from build123d import *

# Parameters (mm, degrees)
SKETCH1_W           = 12.950156288
SKETCH1_H           = 2.985631362
BOSS_EXTRUDE1_DEPTH = 16
FILLET1_R           = 1
SKETCH2_W           = 10.950156288
SKETCH2_H           = 0.272417851
BOSS_EXTRUDE2_DEPTH = 0.1
FILLET2_R           = 0.1
CUT_EXTRUDE2_DEPTH  = 0.1
SKETCH6_W           = 1.186627285
SKETCH6_H           = 15.441785482
SKETCH6_W_2         = 1.175471446
SKETCH6_W_3         = 1.281551352
CUT_EXTRUDE3_DEPTH  = 0.1
SKETCH10_W          = 1.186627285
SKETCH10_H          = 15.441785482
SKETCH10_W_2        = 1.175471446
SKETCH10_W_3        = 1.281551352
CUT_EXTRUDE4_DEPTH  = 0.1
FILLET6_R           = 0.1
FILLET7_R           = 0.1


with BuildPart() as part:
    # Sketch1 → Boss-Extrude1 (new body)
    with BuildSketch(Plane(origin=(0, 0, 0), x_dir=(1, 0, 0), z_dir=(0, 1, 0))):
        Rectangle(SKETCH1_W, SKETCH1_H)
    extrude(amount=BOSS_EXTRUDE1_DEPTH)

    # Fillet1
    fillet1_edges = [part.edges().sort_by_distance(p)[0] for p in [
        (6.475078144, 8, 1.492815681),
        (-6.475078144, 8, 1.492815681),
        (-6.475078144, 8, -1.492815681),
        (6.475078144, 8, -1.492815681),
    ]]
    fillet(fillet1_edges, radius=FILLET1_R)

    # Sketch2 → Boss-Extrude2 (add)
    with BuildSketch(Plane(origin=(0, 0, -1.492815681), x_dir=(-1, 0, 0), z_dir=(0, 0, -1))):
        with Locations((0, 10.703223293)):
            Rectangle(SKETCH2_W, SKETCH2_H)
    extrude(amount=BOSS_EXTRUDE2_DEPTH)

    # Fillet2
    fillet2_edges = [part.edges().sort_by_distance(p)[0] for p in [
        (0, 10.839432218, -1.592815681),
        (-5.475078144, 10.703223292, -1.592815681),
        (0, 10.567014367, -1.592815681),
        (5.475078144, 10.703223292, -1.592815681),
    ]]
    fillet(fillet2_edges, radius=FILLET2_R - 0.0001)  # a hair under: the kernel refuses the full size

    # Sketch5 → Cut-Extrude2 (cut)
    with BuildSketch(Plane(origin=(0, 0, -1.592815681), x_dir=(-1, 0, 0), z_dir=(0, 0, -1))):
        Polygon((-5.375078144, 10.567014367), (5.475078144, 10.567014367), (5.475078144, 10.739432218), (5.475078144, 10.839432218), (-5.375078144, 10.839432218), (-5.475078144, 10.839432218), (-5.475078144, 10.567014367), align=None)
    extrude(amount=-CUT_EXTRUDE2_DEPTH, mode=Mode.SUBTRACT)

    # Sketch6 → Cut-Extrude3 (cut)
    with BuildSketch(Plane(origin=(0, 0, -1.492815681), x_dir=(-1, 0, 0), z_dir=(0, 0, -1))):
        with Locations((-2.737539072, 8)):
            Rectangle(SKETCH6_W, SKETCH6_H)
        with Locations((0, 8)):
            Rectangle(SKETCH6_W_2, SKETCH6_H)
        with Locations((2.737539072, 8)):
            Rectangle(SKETCH6_W_3, SKETCH6_H)
    extrude(amount=-CUT_EXTRUDE3_DEPTH, mode=Mode.SUBTRACT)

    # Sketch10 → Cut-Extrude4 (cut)
    with BuildSketch(Plane.XY.offset(1.492815681)):
        with Locations((2.737539072, 8)):
            Rectangle(SKETCH10_W, SKETCH10_H)
        with Locations((0, 8)):
            Rectangle(SKETCH10_W_2, SKETCH10_H)
        with Locations((-2.737539072, 8)):
            Rectangle(SKETCH10_W_3, SKETCH10_H)
    extrude(amount=-CUT_EXTRUDE4_DEPTH, mode=Mode.SUBTRACT)

    # Fillet6
    fillet6_edges = [part.edges().sort_by_distance(p)[0] for p in [
        (2.144225429, 8, 1.392815681),
        (2.737539072, 15.720892741, 1.392815681),
        (3.330852714, 8, 1.392815681),
        (2.737539072, 0.279107259, 1.392815681),
        (-0.587735723, 8, 1.392815681),
        (0, 15.720892741, 1.392815681),
        (0.587735723, 8, 1.392815681),
        (0, 0.279107259, 1.392815681),
        (-3.378314748, 8, 1.392815681),
        (-2.737539072, 15.720892741, 1.392815681),
        (-2.096763396, 8, 1.392815681),
        (-2.737539072, 0.279107259, 1.392815681),
    ]]
    fillet(fillet6_edges, radius=FILLET6_R - 0.0001)  # a hair under: the kernel refuses the full size

    # Fillet7
    fillet7_edges = [part.edges().sort_by_distance(p)[0] for p in [
        (-3.378314748, 8, -1.392815681),
        (-2.737539072, 0.279107259, -1.392815681),
        (-2.096763396, 8, -1.392815681),
        (-2.737539072, 15.720892741, -1.392815681),
        (-0.587735723, 8, -1.392815681),
        (0, 0.279107259, -1.392815681),
        (0.587735723, 8, -1.392815681),
        (0, 15.720892741, -1.392815681),
        (2.144225429, 8, -1.392815681),
        (2.737539072, 0.279107259, -1.392815681),
        (3.330852714, 8, -1.392815681),
        (2.737539072, 15.720892741, -1.392815681),
    ]]
    fillet(fillet7_edges, radius=FILLET7_R - 0.0001)  # a hair under: the kernel refuses the full size


solid = part.part
Verification items for the finished model (mm, model axes). A direction names the side the tool comes from. Round coordinates to 2 decimals unless told otherwise and drop trailing zeros. Use a Markdown table: item, result. Add a question column.
1. Release check for a two-part mould opening along Y. For faces 4 (the face through (6.475, 8, 0)), 5 (the face through (-3, 8, -1.393)), 6 (the face through (0, 16, 0)) record: released by +Y, released by -Y, zero draft, split by the parting line, or undercut.
2. Thickness scan on probe 1 along Z at (x, y) = (0, 12.75); probe 2 along X at (y, z) = (8.25, -0.55); probe 3 along X at (y, z) = (11, 1.25). Record the ranges inside material, lowest first. Write a range as [from, to].
3. Access from +Z, -Z, +X, -X, +Y, -Y to the whole of each face (thin tool, end or side, straight path). Record for faces 1 (the face through (-3, 8, 1.393)), 2 (the face through (1, 8, 1.493)), 3 (the face through (3, 8, -1.393)).
4. Gauge pin test, flat end, axial feed: pin 1 (0.8 mm diameter, centred on x = 0, y = 9, fed in from -Z). Record the tip position at first contact, or that the pin passes through.
Checks:
| question | item | result |
|---|---|---|
| 1 | face 4 | zero draft |
| 1 | face 5 | undercut |
| 1 | face 6 | released by +Y |
| 2 | probe 1 | z = [-1.39, 1.39] |
| 2 | probe 2 | x = [-6.47, 6.47] |
| 2 | probe 3 | x = [-6.13, 6.13] |
| 3 | face 1 | +Z |
| 3 | face 2 | +Z, +X, -X, +Y, -Y |
| 3 | face 3 | -Z |
| 4 | pin 1 | stops at z = -1.39 |
